Here's how the part is built. I have some questions about the finished solid (model axes, mm). Face numbers are marked on the shaded views. A direction names the side the tool comes from. Give positions to 0.01 mm unless a question says otherwise; leave off trailing zeros. Loops run counter-clockwise (first coordinate to the right, second up) from the corner with the lowest first, then second, coordinate; pieces in that order, holes last. Notation, with made-up numbers: (27, 71) - (39, 71) arc R22 cw to (39, 94) - close; hole circle Ø8 at (-11, 57.5). An arc over 180 degrees is marked (long way). Use one line per item in the form item = value.
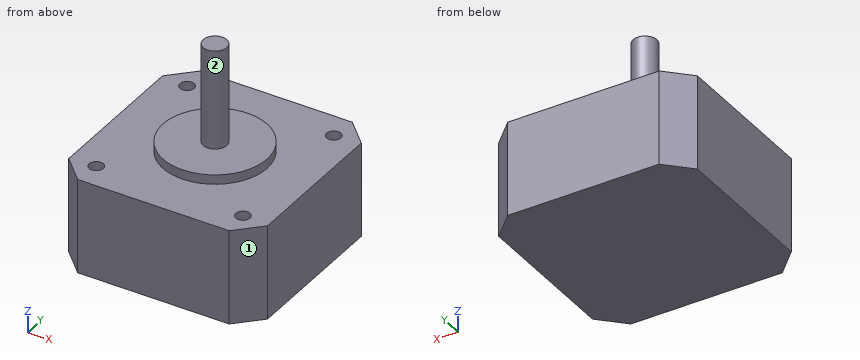
from build123d import *

# Parameters (mm, degrees)
F0_W     = 42
F0_H     = 42
F1_DEPTH = 20
F2_R     = 11
F3_DEPTH = 2
F4_R     = 2.5
F5_DEPTH = 21
F6_R     = 1.5
F7_DEPTH = 4.5
F8_SIZE  = 5


with BuildPart() as f1:
    # F0 (on Top) → F1 (new body)
    with BuildSketch(Plane.XY):
        Rectangle(F0_W, F0_H)
    extrude(amount=F1_DEPTH)

    # F2 (on face) → F3 (join)
    with BuildSketch(Plane.XY.offset(20)):
        Circle(F2_R)
    extrude(amount=F3_DEPTH)

    # F4 (on face) → F5 (join)
    with BuildSketch(Plane.XY.offset(22)):
        Circle(F4_R)
    extrude(amount=F5_DEPTH)

    # F6 (on face) → F7 (cut)
    with BuildSketch(Plane.XY.offset(20)):
        with Locations((-15.5, 15.5)):
            Circle(F6_R)
        with Locations((-15.5, -15.5)):
            Circle(F6_R)
        with Locations((15.5, 15.5)):
            Circle(F6_R)
        with Locations((15.5, -15.5)):
            Circle(F6_R)
    extrude(amount=-F7_DEPTH, mode=Mode.SUBTRACT)

    # F8
    f8_edges = [f1.edges().sort_by_distance(p)[0] for p in [
        (21, 21, 10),
        (21, -21, 10),
        (-21, -21, 10),
        (-21, 21, 10),
    ]]
    chamfer(f8_edges, length=F8_SIZE)


solid = f1.part
(1) For the marked faces 1 and 2, which set-ups out of +Z, -Z, +X, -X, +Y, -Y let a thin tool reach every point of the face, with its end or its side?
Geometry says:
face_1 = +Z, -Z, +X, -Y
face_2 = +Z
(2) If we section it at D-D (x = 8): List the corners of the cut face in (y, z) for me.
Geometry says:
outline = (-21, 0) - (21, 0) - (21, 20) - (7.55, 20) - (7.55, 22) - (-7.55, 22) - (-7.55, 20) - (-21, 20) - close
(3) If we section it at A-A (x = 0): List the corners of the cut face in (y, z) for me, plus the area to 3 significant figures.
Geometry says:
outline = (-21, 0) - (21, 0) - (21, 20) - (11, 20) - (11, 22) - (2.5, 22) - (2.5, 43) - (-2.5, 43) - (-2.5, 22) - (-11, 22) - (-11, 20) - (-21, 20) - close
area = 989 mm²
(4) If we section it at B-B (z = 12): List the corners of the cut face in (x, y) for me.
Geometry says:
outline = (-21, -16) - (-16, -21) - (16, -21) - (21, -16) - (21, 16) - (16, 21) - (-16, 21) - (-21, 16) - close
(5) For P1, Ø1, axis at x = -1, y = 15.5, coming from the +Z side; P2, Ø0.9, axis at x = -15.5, y = -15.5, coming from the +Z side; P3, Ø12.5, axis at x = -8, y = -5, coming from the +Z side, each with a flat end and sliding along its axis, tell me the tip position at first contact or that it passes through.
Geometry says:
P1 = 20
P2 = 15.5
P3 = 22
(6) If we section it at C-C (y = 1.5): List the corners of the cut face in (x, z) for me.
Geometry says:
outline = (-21, 0) - (21, 0) - (21, 20) - (10.9, 20) - (10.9, 22) - (2, 22) - (2, 43) - (-2, 43) - (-2, 22) - (-10.9, 22) - (-10.9, 20) - (-21, 20) - close
(7) If I drill on probe 1 along Y at (x, z) = (15.5, 16.95); probe 2 along Y at (x, z) = (-15, 18); probe 3 along Z at (x, y) = (17, -7.5), over which ranges is the centre line in solid material (lowest first)?
Geometry says:
probe_1 = -21 to -17, -14 to 14, 17 to 21
probe_2 = -21 to -16.91, -14.09 to 14.09, 16.91 to 21
probe_3 = 0 to 20
